```python
from build123d import *

# Parameters (mm, degrees)
SCHIZZO1_R                   = 15
ESTRUSIONE_ESTRUSIONE1_DEPTH = 50
SCHIZZO2_R                   = 8
ESTRUSIONE_ESTRUSIONE2_DEPTH = 15
ESTRUSIONE_ESTRUSIONE3_DEPTH = 10


with BuildPart() as part:
    # Schizzo1 → Estrusione-Estrusione1 (new body)
    with BuildSketch(Plane.XY):
        Circle(SCHIZZO1_R)
    extrude(amount=ESTRUSIONE_ESTRUSIONE1_DEPTH)

    # Schizzo2 → Estrusione-Estrusione2 (add)
    with BuildSketch(Plane.XY.offset(50)):
        Circle(SCHIZZO2_R)
    extrude(amount=ESTRUSIONE_ESTRUSIONE2_DEPTH)

    # Schizzo3 → Estrusione-Estrusione3 (add)
    with BuildSketch(Plane(origin=(0, 0, 0), x_dir=(-1, 0, 0), z_dir=(0, 0, -1))):
        Polygon((10, 0), (5, 8.660254038), (-5, 8.660254038), (-10, 0), (-5, -8.660254038), (5, -8.660254038), align=None)
    extrude(amount=ESTRUSIONE_ESTRUSIONE3_DEPTH)


solid = part.part
```
For this review, take the finished solid that the model builds, in its own axes (mm). A direction names the side the tool comes from. Round coordinates to 2 decimals unless told otherwise and drop trailing zeros. Write each loop counter-clockwise with the first axis right and the second up, starting at its lowest first coordinate (ties: lowest second). Pieces come first, ordered by that corner, then holes. Notation, with made-up numbers: (51, 16) -> (107, 16) arc R17 ccw to (107, 41) -> close; hole circle Ø11 at (-36, -38). An arc over 180 degrees is marked (long way). Use one line per item in the form item = value.
Q1. Machinability: for faces 1 (the flat face through (0, 8.66, -5)), 2 (the flat face through (-7.535, 4.27, -4.93)), 3 (the flat face through (7.535, -4.27, -4.93)), which of the approach directions +Z, -Z, +X, -X, +Y, -Y give a long, thin tool a straight path to every point of the face, cutting with its end or side? Answer none if there is none.
Resolved:
face_1 = -Z, +X, -X, +Y
face_2 = -Z, -X, +Y
face_3 = -Z, +X, -Y
Q2. Consider section C-C (y = -4.5). State the section outline as (x, z) points.
Resolved:
outline = (-14.31, 0) -> (-7.4, 0) -> (-7.4, -10) -> (7.4, -10) -> (7.4, 0) -> (14.31, 0) -> (14.31, 50) -> (6.61, 50) -> (6.61, 65) -> (-6.61, 65) -> (-6.61, 50) -> (-14.31, 50) -> close
Q3. Consider section B-B (z = 59). State the section outline as (x, y) points.
Resolved:
outline = circle Ø16 at (0, 0)
Q4. Clearance check with flat-ended pins moving along their axes: pin 1 Ø2 at (y, z) = (6.5, 15) entering from -X; pin 2 Ø6 at (y, z) = (0.5, 34.5) entering from +X; pin 3 Ø1.5 at (x, z) = (8, 41) entering from +Y; pin 4 Ø4 at (y, z) = (11.5, 26.5) entering from -X. State where each tip first meets the part, or that it passes through.
Resolved:
pin_1 = -13.96
pin_2 = 15
pin_3 = 13.13
pin_4 = -11.61
Q5. To check wall thickness, follow probe 1 along Z at (x, y) = (4.5, 11.5); probe 2 along Y at (x, z) = (-4.75, 21.5). State the ranges of each line that lie inside material, in increasing order. Write a range as from..to.
Resolved:
probe_1 = 0..50
probe_2 = -14.23..14.23
Q6. Consider section A-A (x = 0). State the section outline as (y, z) points, then the cut area to 3 significant figures.
Resolved:
outline = (-15, 0) -> (-8.66, 0) -> (-8.66, -10) -> (8.66, -10) -> (8.66, 0) -> (15, 0) -> (15, 50) -> (8, 50) -> (8, 65) -> (-8, 65) -> (-8, 50) -> (-15, 50) -> close
area = 1,910 mm²
Q7. Consider section D-D (x = -10.75). State the section outline as (y, z) points.
Resolved:
outline = (-10.46, 0) -> (10.46, 0) -> (10.46, 50) -> (-10.46, 50) -> close
